```python
from build123d import *

# Parameters (mm, degrees)
SKETCH1_R    = 2
SHAFT_DEPTH  = 12
SKETCH2_R    = 12.5
BODY_DEPTH   = 75
SKETCH3_W    = 3
SKETCH3_H    = 6
D_FLAT_DEPTH = 10


with BuildPart() as part:
    # Sketch1 → Shaft (new body)
    with BuildSketch(Plane.XY):
        Circle(SKETCH1_R)
    extrude(amount=SHAFT_DEPTH)

    # Sketch2 → Body (add)
    with BuildSketch(Plane.XY.offset(12)):
        Circle(SKETCH2_R)
    extrude(amount=BODY_DEPTH)

    # Sketch3 → D_flat (cut)
    with BuildSketch(Plane.XY):
        with Locations((3, 0)):
            Rectangle(SKETCH3_W, SKETCH3_H)
    extrude(amount=D_FLAT_DEPTH, mode=Mode.SUBTRACT)


solid = part.part
```
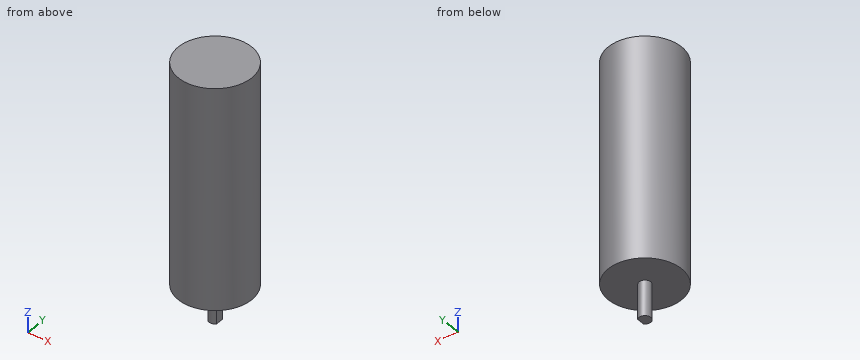
Could you check a few things on this model? Use its own coordinates, in mm. Round coordinates to 2 decimals unless told otherwise and drop trailing zeros. Write each loop counter-clockwise with the first axis right and the second up, starting at its lowest first coordinate (ties: lowest second). Pieces come first, ordered by that corner, then holes.
(1) Suppose I cut it at B-B on y = 3.5. Write out the boundary of the cut face in (x, z).
Findings below:
outline: (-12, 12) - (12, 12) - (12, 87) - (-12, 87) - close
(2) If I drill on probe 1 along Z at (x, y) = (-3, 9.25); probe 2 along Y at (x, z) = (0.25, 16), over which ranges is the centre line in solid material (lowest first)?
Findings below:
probe 1: z = 12 to 87
probe 2: y = -12.5 to 12.5
(3) Suppose I cut it at A-A on x = 0. Write out the boundary of the cut face in (y, z), and give its area (3 significant figures).
Findings below:
outline: (-12.5, 12) - (-2, 12) - (-2, 0) - (2, 0) - (2, 12) - (12.5, 12) - (12.5, 87) - (-12.5, 87) - close
area: 1,920 mm2
(4) Suppose I cut it at C-C on z = 16.5. Write out the boundary of the cut face in (x, y).
Findings below:
outline: circle Ø25 at (0, 0)
(5) For pin 1 (12.5 mm diameter, centred on x = -5, y = 5.5, fed in from -Z); pin 2 (1.5 mm diameter, centred on x = 3.5, z = 23, fed in from -Y); pin 3 (8 mm diameter, centred on y = -5, z = 32, fed in from -X); pin 4 (4 mm diameter, centred on x = 5, y = 0.5, fed in from -Z), each with a flat end and sliding along its axis, tell me the tip position at first contact or that it passes through.
Findings below:
pin 1: stops at z = 0
pin 2: stops at y = -12.19
pin 3: stops at x = -12.46
pin 4: stops at z = 12
(6) Suppose I cut it at D-D on x = 5.25. Write out the boundary of the cut face in (y, z).
Findings below:
outline: (-11.34, 12) - (11.34, 12) - (11.34, 87) - (-11.34, 87) - close
